from build123d import *

# Parameters (mm, degrees)
SKETCH1_W           = 101.6
SKETCH1_H           = 12.7
BOSS_EXTRUDE1_DEPTH = 12.7
SKETCH2_R           = 3.429
CUT_EXTRUDE1_DEPTH  = 54.881536726
CUT_EXTRUDE2_DEPTH  = 2.794


with BuildPart() as part:
    # Sketch1 → Boss-Extrude1 (new body)
    with BuildSketch(Plane(origin=(0, 0, 0), x_dir=(1, 0, 0), z_dir=(0, 1, 0))):
        with Locations((0, 6.35)):
            Rectangle(SKETCH1_W, SKETCH1_H)
    extrude(amount=BOSS_EXTRUDE1_DEPTH)

    # Sketch2 → Cut-Extrude1 (cut, through all)
    with BuildSketch(Plane(origin=(0, 12.7, 0), x_dir=(1, 0, 0), z_dir=(0, 1, 0))):
        with Locations(Location((-38.1, 6.35, 0), (0, 0, 270))):
            Circle(SKETCH2_R)
        with Locations(Location((38.1, 6.35, 0), (0, 0, 270))):
            Circle(SKETCH2_R)
        with Locations(Location((-12.7, 6.35, 0), (0, 0, 270))):
            Circle(SKETCH2_R)
        with Locations(Location((12.7, 6.35, 0), (0, 0, 270))):
            Circle(SKETCH2_R)
    extrude(amount=-CUT_EXTRUDE1_DEPTH, mode=Mode.SUBTRACT)

    # Sketch3 → Cut-Extrude2 (cut, symmetric)
    with BuildSketch(Plane(origin=(0, 6.35, 0), x_dir=(1, 0, 0), z_dir=(0, 1, 0))):
        Polygon((-18.161, 3.19709018), (-18.161, 19.396139053), (-7.239, 19.396139053), (-7.239, 9.50290982), (-7.239, 3.19709018), (-12.7, 0.04418036), align=None)
        Polygon((7.239, 19.396139053), (18.161, 19.396139053), (18.161, 9.50290982), (18.161, 3.19709018), (12.7, 0.04418036), (7.239, 3.19709018), align=None)
    extrude(amount=CUT_EXTRUDE2_DEPTH, both=True, mode=Mode.SUBTRACT)


solid = part.part
Input: part model. Units: mm. Frame: model coordinates. A direction names the side the tool comes from. Coordinates: 2 decimals unless noted, no trailing zeros. Loops run counter-clockwise (first coordinate to the right, second up) from the corner with the lowest first, then second, coordinate; pieces in that order, holes last. Notation, with made-up numbers: (3, -21.75) -> (53, -21.75) arc R28 cw to (53, 1.25) -> close; hole circle Ø3 at (67.5, 68). An arc over 180 degrees is marked (long way). One line per item, written item: value.
(1) Cut plane A-A (y = 8). Output: boundary loops of the cut face in (x, z).
Answer below:
outline: (-50.8, -12.7) -> (-18.16, -12.7) -> (-18.16, -3.2) -> (-12.7, -0.04) -> (-7.24, -3.2) -> (-7.24, -12.7) -> (7.24, -12.7) -> (7.24, -3.2) -> (12.7, -0.04) -> (18.16, -3.2) -> (18.16, -12.7) -> (50.8, -12.7) -> (50.8, 0) -> (-50.8, 0) -> close; hole circle Ø6.86 at (-38.1, -6.35); hole circle Ø6.86 at (38.1, -6.35)
(2) Cut plane C-C (z = -6.35). Give the number of separate pieces and of enclosed holes in the cut face, then the cut area to 3 significant figures.
Answer below:
separate pieces: 5
enclosed holes: 0
area: 897 mm2
(3) Ray query, line 1 along X through (y, z) = (1.3, -6.35); line 2 along X through (y, z) = (6, -10.5); line 3 along X through (y, z) = (5, -6.35). Return the intervals inside material, ascending.
Answer below:
line 1: x = -50.8 to -41.53, -34.67 to -16.13, -9.27 to 9.27, 16.13 to 34.67, 41.53 to 50.8
line 2: x = -50.8 to -18.16, -7.24 to 7.24, 18.16 to 50.8
line 3: x = -50.8 to -41.53, -34.67 to -18.16, -7.24 to 7.24, 18.16 to 34.67, 41.53 to 50.8
(4) Cut plane D-D (x = -11). Output: boundary loops of the cut face in (y, z).
Answer below:
outline: (0, -12.7) -> (3.56, -12.7) -> (3.56, -9.33) -> (0, -9.33) -> close; (0, -3.37) -> (3.56, -3.37) -> (3.56, -1.03) -> (9.14, -1.03) -> (9.14, -3.37) -> (12.7, -3.37) -> (12.7, 0) -> (0, 0) -> close; (9.14, -12.7) -> (12.7, -12.7) -> (12.7, -9.33) -> (9.14, -9.33) -> close
(5) Cut plane B-B (x = -38.1). Output: boundary loops of the cut face in (y, z), then the cut area to 3 significant figures.
Answer below:
outline: (0, -12.7) -> (12.7, -12.7) -> (12.7, -9.78) -> (0, -9.78) -> close; (0, -2.92) -> (12.7, -2.92) -> (12.7, 0) -> (0, 0) -> close
area: 74.2 mm2
(6) Draft query along Z for faces 1 (the face through (10.008, 6.389, -1.599)), 2 (the face through (-14.01, 1.8, -3.18)), 3 (the face through (-34.7, 6.4, -6.8)), 4 (the face through (50.8, 6, -6)). Return one class per face: pulls with the +Z half, pulls with the -Z half, needs draft (parallel to the pull), parting line crosses it, or undercut.
Answer below:
face 1: pulls with the -Z half
face 2: undercut
face 3: undercut
face 4: needs draft
(7) Set-up query: faces 5 (the face through (-1, 6, -12.7)), 6 (the face through (-15.1, 9.144, -9.3)). Return all of +Z, -Z, +X, -X, +Y, -Y with unobstructed straight access to the full face (end or side cutting, diameter ignored); none if empty.
Answer below:
face 5: -Z, +X, -X, +Y, -Y
face 6: -Z
